```python
from build123d import *

# Parameters (mm, degrees)
SKETCH3_R             = 5
CUT_EXTRUDE1_DEPTH    = 167.770800802
F_8_0MM_DOWEL_HOLE1_D = 8
CIRPATTERN1_COUNT     = 18
SKETCH7_R             = 2.65
CUT_EXTRUDE2_DEPTH    = 163.903345576
CIRPATTERN2_COUNT     = 15


with BuildPart() as part:
    # Sketch1 → Revolve1 (revolve)
    with BuildSketch(Plane.XY, mode=Mode.PRIVATE) as revolve1_sk:
        Polygon((0, 112.5), (0, 80), (15, 80), (15, 98.5), (50, 98.5), (50, 112.5), align=None)
    revolve(revolve1_sk.sketch.rotate(Axis((0, 0, 0), (1, 0, 0)), 90), axis=Axis((0, 0, 0), (1, 0, 0)))

    # Sketch3 → Cut-Extrude1 (cut, through all)
    with BuildSketch(Plane(origin=(50, 0, 0), x_dir=(0, 0, -1), z_dir=(1, 0, 0))):
        with Locations((105.5, 0)):
            Circle(SKETCH3_R)
        with Locations(Location((-105.5, 0, 0), (0, 0, 180))):
            Circle(SKETCH3_R)
    extrude(amount=-CUT_EXTRUDE1_DEPTH, mode=Mode.SUBTRACT)

    # 8.0mm Dowel Hole1 (through all)
    with Locations(Plane(origin=(50, 105.5, 0), x_dir=(0, 0, 1), z_dir=(1, 0, 0))):
        with Locations((0, 0)):
            f_8_0mm_dowel_hole1 = Hole(F_8_0MM_DOWEL_HOLE1_D / 2)

    # CirPattern1: 8.0mm Dowel Hole1 ×18 about axis
    cirpattern1_axis = Axis((0, 0, 0), (1, 0, 0))
    for i in range(1, CIRPATTERN1_COUNT):
        add(f_8_0mm_dowel_hole1.rotate(cirpattern1_axis, i * 360 / CIRPATTERN1_COUNT), mode=Mode.SUBTRACT)

    # Sketch7 → Cut-Extrude2 (cut, through all)
    with BuildSketch(Plane(origin=(15, 0, 0), x_dir=(0, 0, -1), z_dir=(1, 0, 0))):
        with Locations((87.75, 0)):
            Circle(SKETCH7_R)
    cut_extrude2 = extrude(amount=-CUT_EXTRUDE2_DEPTH, mode=Mode.SUBTRACT)

    # CirPattern2: Cut-Extrude2 ×15 about axis
    cirpattern2_axis = Axis((0, 0, 0), (1, 0, 0))
    for i in range(1, CIRPATTERN2_COUNT):
        add(cut_extrude2.rotate(cirpattern2_axis, i * 360 / CIRPATTERN2_COUNT), mode=Mode.SUBTRACT)


solid = part.part
```
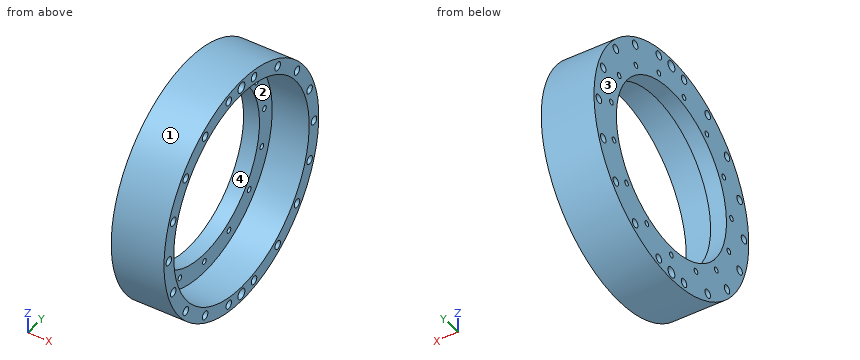
Geometry: final body of the model. Coordinates: model frame, mm. Face numbers are marked on the shaded views. Give positions to 0.01 mm unless a question says otherwise; leave off trailing zeros. Loops run counter-clockwise (first coordinate to the right, second up) from the corner with the lowest first, then second, coordinate; pieces in that order, holes last. Notation, with made-up numbers: (55, 0.25) -> (110, 0.25) arc R17 cw to (110, 14.25) -> close; hole circle Ø2 at (87.5, 14). An arc over 180 degrees is marked (long way). Return JSON: item names as keys, results as strings.
Item 1: Mould query, pull axis Y, two halves, no side actions, for the marked faces 1, 2, 3 and 4. Classes: released by +Y, released by -Y, zero draft, split by the parting line, or undercut.
Filled in:
{"face 1": "split by the parting line", "face 2": "undercut", "face 3": "zero draft", "face 4": "undercut"}
Item 2: Section B-B, the plane x = 40.5. Count the separate pieces of the cut face and the enclosed holes in it, plus the area to 3 significant figures.
Filled in:
{"separate pieces": "1", "enclosed holes": "21", "area": "8,220 mm^2"}
Item 3: Section C-C, the plane z = -37. Output: boundary loops of the cut face in (x, y).
Filled in:
{"outline": "(0, -106.24) -> (50, -106.24) -> (50, -103.03) -> (0, -103.03) -> close; (0, -95.24) -> (50, -95.24) -> (50, -91.29) -> (15, -91.29) -> (15, -70.93) -> (0, -70.93) -> close; (0, 70.93) -> (15, 70.93) -> (15, 91.29) -> (50, 91.29) -> (50, 95.24) -> (0, 95.24) -> close; (0, 103.03) -> (50, 103.03) -> (50, 106.24) -> (0, 106.24) -> close"}
Item 4: Section A-A, the plane z = 0. Output: boundary loops of the cut face in (x, y), plus the area to 4 significant figures.
Filled in:
{"outline": "(0, -112.5) -> (50, -112.5) -> (50, -109.5) -> (0, -109.5) -> close; (0, -101.5) -> (50, -101.5) -> (50, -98.5) -> (15, -98.5) -> (15, -80) -> (0, -80) -> close; (0, 80) -> (15, 80) -> (15, 98.5) -> (50, 98.5) -> (50, 101.5) -> (0, 101.5) -> close; (0, 109.5) -> (50, 109.5) -> (50, 112.5) -> (0, 112.5) -> close", "area": "1,155 mm^2"}
Item 5: Pin query (flat end, axial travel): P1, Ø12, axis at x = 15.5, z = 42, coming from the +Y side; P2, Ø7, axis at y = 75.99, z = 43.87, coming from the +X side; P3, Ø3, axis at x = 5, z = -41, coming from the -Y side. Return the tip coordinate at first contact, or that it passes through.
Filled in:
{"P1": "y = 106.58", "P2": "x = 15", "P3": "y = -105.34"}
Item 6: Line query: line 1 (Y direction, x = 8.5, z = 102.5); line 2 (Y direction, x = 26, z = 0); line 3 (Z direction, x = 13, y = -18.5). Output: solid intervals per line, ascending.
Filled in:
{"line 1": "-46.37 to -22.07, -14.57 to -4, 4 to 14.57, 22.07 to 46.37", "line 2": "-112.5 to -109.5, -101.5 to -98.5, 98.5 to 101.5, 109.5 to 112.5", "line 3": "-110.97 to -107.89, -99.9 to -77.83, 77.83 to 83.19, 88.47 to 99.9, 107.89 to 110.97"}
